Source: CAD feature listing. Evaluate the final solid. Frame: model axes, mm. Face numbers are marked on the shaded views. A direction names the side the tool comes from. Round coordinates to 2 decimals unless told otherwise and drop trailing zeros. Order: outer loops, then holes, each group sorted by start corner. A loop starts at its lowest first (then second) coordinate and runs counter-clockwise, first axis right, second up. Notation, with made-up numbers: M 83.25,6.25 L 101.25,6.25 A26 ccw 101.25,25.25 Z; hole C 30.25,18.5 d11. An arc over 180 degrees is marked long. Answer as CSV lines item,"result". Start each with the question number.
Item 1: Set-up query: the marked faces 1, 2, 3 and 4. Return all of +Z, -Z, +X, -X, +Y, -Y with unobstructed straight access to the full face (end or side cutting, diameter ignored); none if empty.
Item 2: Section query B-B on x = 0. Return the cut outline in (y, z).
Item 3: Section query C-C on y = 16. Return the cut outline in (x, z).
Item 4: Section query A-A on z = 0. Return the cut outline in (x, y), plus the area to 3 significant figures.
Item 5: First-contact query: P1, Ø1.6, axis at x = 0, z = 0, coming from the +Y side; P2, Ø1.5, axis at y = 11, z = 1.5, coming from the +X side. Flat tips, straight axial feed; report the tip coordinate or a pass-through.
Item 6: Line query: line 1 (Y direction, x = 1, z = -1.25); line 2 (X direction, y = 18.5, z = 0). Output: solid intervals per line, ascending. Write a range as [from, to].
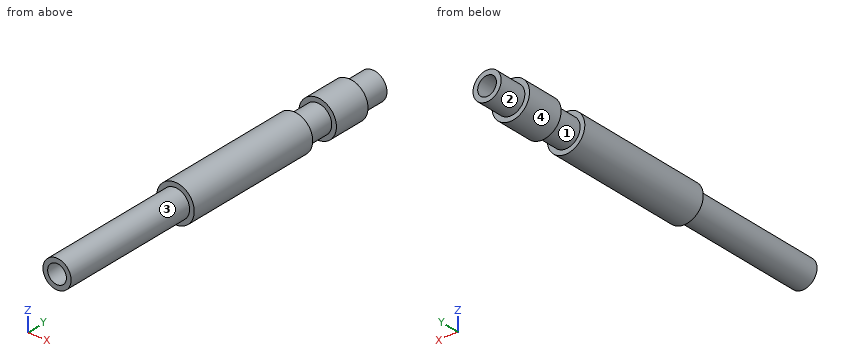
from build123d import *

# Parameters (mm, degrees)
SKETCH_1_R      = 2
SKETCH_1_R_2    = 1
EXTRUDE_1_DEPTH = 40
SKETCH_2_W      = 0.5
SKETCH_2_H      = 3
SKETCH_3_W      = 0.5
SKETCH_3_H      = 15


with BuildPart() as part:
    # Эскиз1 → Бобышка-Вытянуть1 (new body)
    with BuildSketch(Plane(origin=(0, 0, 0), x_dir=(1, 0, 0), z_dir=(0, 1, 0))):
        Circle(SKETCH_1_R)
        Circle(SKETCH_1_R_2, mode=Mode.SUBTRACT)
    extrude(amount=EXTRUDE_1_DEPTH)

    # Эскиз2 → Вырез-Повернуть1 (revolve, cut)
    with BuildSketch(Plane.XY):
        with Locations((1.75, 38.5)):
            Rectangle(SKETCH_2_W, SKETCH_2_H)
        with Locations((1.75, 31.5)):
            Rectangle(SKETCH_2_W, SKETCH_2_H)
    revolve(axis=Axis((0, 40, 0), (0, -1, 0)), mode=Mode.SUBTRACT)

    # Эскиз3 → Вырез-Повернуть2 (revolve, cut)
    with BuildSketch(Plane.XY):
        with Locations((1.75, 7.5)):
            Rectangle(SKETCH_3_W, SKETCH_3_H)
    revolve(axis=Axis((0, 0, 0), (0, 1, 0)), mode=Mode.SUBTRACT)


solid = part.part
Results:
1,face 1,"none"
1,face 2,"+Y"
1,face 3,"-Y"
1,face 4,"+Y, -Y"
2,outline,"M 0,-1.5 L 15,-1.5 L 15,-2 L 30,-2 L 30,-1.5 L 33,-1.5 L 33,-2 L 37,-2 L 37,-1.5 L 40,-1.5 L 40,-1 L 0,-1 Z; M 0,1 L 40,1 L 40,1.5 L 37,1.5 L 37,2 L 33,2 L 33,1.5 L 30,1.5 L 30,2 L 15,2 L 15,1.5 L 0,1.5 Z"
3,outline,"C 0,0 d4; hole C 0,0 d2"
4,outline,"M -2,15 L -1.5,15 L -1.5,0 L -1,0 L -1,40 L -1.5,40 L -1.5,37 L -2,37 L -2,33 L -1.5,33 L -1.5,30 L -2,30 Z; M 1,0 L 1.5,0 L 1.5,15 L 2,15 L 2,30 L 1.5,30 L 1.5,33 L 2,33 L 2,37 L 1.5,37 L 1.5,40 L 1,40 Z"
4,area,"59.0 mm^2"
5,P1,"through"
5,P2,"x = 1.3"
6,line 1,"[15, 30], [33, 37]"
6,line 2,"[-2, -1], [1, 2]"
